Read the model definition and answer for the solid it produces. Units are mm, in the model's axes. A direction names the side the tool comes from. Round coordinates to 2 decimals unless told otherwise and drop trailing zeros. Use one line per item in the form item = value. Start each with the question number.
from build123d import *

# Parameters (mm, degrees)
F0_R          = 2.125
F0_R_2        = 5.25
F1_DEPTH      = 5
F3_DEPTH      = 15
F4_R          = 2.125
F5_DEPTH      = 25
F6_W          = 50
F6_H          = 15
F6_R          = 2.125
F7_DEPTH      = 5
F8_R          = 7.5
F9_SIZE       = 7.5
F10_R         = 2.125
F10_R_2       = 11.5
F11_DEPTH     = 3.75
F12_T1_DEPTH  = 10
F12_T6_DEPTH  = 4
F12_S7_R      = 25
F12_T8_DEPTH  = 4
F12_T12_DEPTH = 4
F12_S13_R     = 25
F12_T14_DEPTH = 4
F13_R         = 4.99999
F14_R         = 1.99999
F15_R         = 5.5
F16_DEPTH     = 25


# Not quite as in the source:
# - a fillet or chamfer that OpenCascade refuses, or shapes differently, is made with other operations: its cross-section is extruded or revolved along the edge and cut away or added
# - a fillet or chamfer is up to 0.001 mm smaller than in the source, because OpenCascade refuses the exact size


with BuildPart() as f1:
    # F0 (on Top) → F1 (new body)
    with BuildSketch(Plane.XY):
        with BuildLine():
            Line((25, -27.1), (25, -22.1))
            Line((25, -22.1), (25, 0))
            ThreePointArc((25, 0), (0, 25), (-25, 0))
            Line((-25, 0), (-25, -22.1))
            Line((-25, -22.1), (-25, -27.1))
            Line((-25, -27.1), (25, -27.1))
        make_face()
        with Locations((-13.8564064606, -8)):
            Circle(F0_R, mode=Mode.SUBTRACT)
        with Locations((13.8564064606, -8)):
            Circle(F0_R, mode=Mode.SUBTRACT)
        Circle(F0_R_2, mode=Mode.SUBTRACT)
        with Locations((0, 16)):
            Circle(F0_R, mode=Mode.SUBTRACT)
    extrude(amount=F1_DEPTH)

    # F2 (on face) → F3 (join)
    with BuildSketch(Plane.XY.offset(5)):
        Polygon((-25, -27.1), (25, -27.1), (25, -22.1), (25, 0), (21, 0), (21, -22.1), (5, -22.1), (5, -14.1), (0, -14.1), (-5, -14.1), (-5, -22.1), (-21, -22.1), (-21, 0), (-25, 0), (-25, -22.1), align=None)
    extrude(amount=F3_DEPTH)

    # F4 (on face) → F5 (cut)
    with BuildSketch(Plane.XZ.offset(27.1)):
        with Locations((-11.725, 12.5)):
            Circle(F4_R)
        with Locations((11.725, 12.5)):
            Circle(F4_R)
    extrude(amount=-F5_DEPTH, mode=Mode.SUBTRACT)

    # F6 (on Top) → F7 (join)
    with BuildSketch(Plane.XY):
        with Locations((0, -34.6)):
            Rectangle(F6_W, F6_H)
        with Locations((-17.5, -34.6)):
            Circle(F6_R, mode=Mode.SUBTRACT)
        with Locations((17.5, -34.6)):
            Circle(F6_R, mode=Mode.SUBTRACT)
    extrude(amount=F7_DEPTH)

    # F8
    f8_edges = [f1.edges().sort_by_distance(p)[0] for p in [
        (-25, -42.1, 2.5),
        (25, -42.1, 2.5),
    ]]
    fillet(f8_edges, radius=F8_R)

    # F9
    f9_edges = [f1.edges().sort_by_distance(p)[0] for p in [
        (0, -14.1, 20),
        (-23, 0, 20),
        (23, 0, 20),
    ]]
    chamfer(f9_edges, length=F9_SIZE)

    # F10 (on face) → F11 (join)
    with BuildSketch(Plane.XY.offset(5)):
        with BuildLine():
            Line((25, -22.1), (25, 0))
            ThreePointArc((25, 0), (0, 25), (-25, 0))
            Line((-25, 0), (-25, -22.1))
            Line((-25, -22.1), (25, -22.1))
        make_face()
        with Locations((-13.8564064606, -8)):
            Circle(F10_R, mode=Mode.SUBTRACT)
        Circle(F10_R_2, mode=Mode.SUBTRACT)
        with Locations((13.8564064606, -8)):
            Circle(F10_R, mode=Mode.SUBTRACT)
        with Locations((0, 16)):
            Circle(F10_R, mode=Mode.SUBTRACT)
    extrude(amount=F11_DEPTH)

    # F12: chamfer of 2.5 on 3 edges, made by hand

    # F12_s2 → F12_t1 (join)
    with BuildSketch(Plane.YZ.offset(-5)):
        with BuildLine():
            Line((-14.1707106781, 11.3207106781), (-11.5292893219, 8.6792893219))
            Line((-11.5292893219, 8.6792893219), (-11.5292893219, 8.6292893219))
            ThreePointArc((-11.5292893219, 8.6292893219), (-12.8146446609, 8.7), (-14.1, 8.7))
            Line((-14.1, 8.7), (-14.15, 8.75))
            ThreePointArc((-14.15, 8.75), (-14.15, 10.0353553391), (-14.2207106781, 11.3207106781))
            Line((-14.2207106781, 11.3207106781), (-14.1707106781, 11.3207106781))
        make_face()
    extrude(amount=F12_T1_DEPTH)


with BuildPart() as f12_tool4:
    # F12_s5 → F12_t6 (new body)
    with BuildSketch(Plane.YZ.offset(-21)):
        with BuildLine():
            Line((-0.0707106781, 11.3207106781), (2.5707106781, 8.6792893219))
            Line((2.5707106781, 8.6792893219), (2.5707106781, 8.6292893219))
            ThreePointArc((2.5707106781, 8.6292893219), (1.2853553391, 8.7), (0, 8.7))
            Line((0, 8.7), (-0.05, 8.75))
            ThreePointArc((-0.05, 8.75), (-0.05, 10.0353553391), (-0.1207106781, 11.3207106781))
            Line((-0.1207106781, 11.3207106781), (-0.0707106781, 11.3207106781))
        make_face()
    extrude(amount=-F12_T6_DEPTH)

    # F12_s7 → F12_t8 (intersect, symmetric)
    with BuildSketch(Plane.XY.offset(10)):
        Circle(F12_S7_R)
    extrude(amount=F12_T8_DEPTH, both=True, mode=Mode.INTERSECT)


with BuildPart() as f1_1:
    add(f1.part)

    # F12_t3: union F12_tool4
    add(f12_tool4.part)


with BuildPart() as f12_tool10:
    # F12_s11 → F12_t12 (new body)
    with BuildSketch(Plane.YZ.offset(25)):
        with BuildLine():
            Line((2.5707106781, 8.6792893219), (-0.0707106781, 11.3207106781))
            Line((-0.0707106781, 11.3207106781), (-0.1207106781, 11.3207106781))
            ThreePointArc((-0.1207106781, 11.3207106781), (-0.05, 10.0353553391), (-0.05, 8.75))
            Line((-0.05, 8.75), (0, 8.7))
            ThreePointArc((0, 8.7), (1.2853553391, 8.7), (2.5707106781, 8.6292893219))
            Line((2.5707106781, 8.6292893219), (2.5707106781, 8.6792893219))
        make_face()
    extrude(amount=-F12_T12_DEPTH)

    # F12_s13 → F12_t14 (intersect, symmetric)
    with BuildSketch(Plane.XY.offset(10)):
        Circle(F12_S13_R)
    extrude(amount=F12_T14_DEPTH, both=True, mode=Mode.INTERSECT)


with BuildPart() as f1_2:
    add(f1_1.part)

    # F12_t9: union F12_tool10
    add(f12_tool10.part)

    # F13 (radius 5 in the source; OpenCascade refuses exactly that, so slightly less here)
    f13_edges = [f1_2.edges().sort_by_distance(p)[0] for p in [
        (5, -17.85, 16.25),
        (-5, -17.85, 16.25),
    ]]
    fillet(f13_edges, radius=F13_R)

    # F14 (radius 2 in the source; OpenCascade refuses exactly that, so slightly less here)
    f14_edges = [f1_2.edges().sort_by_distance(p)[0] for p in [
        (21, -14.8, 20),
        (25, -17.3, 20),
        (-21, -14.8, 20),
        (-25, -17.3, 20),
        (0, 25, 8.75),
    ]]
    fillet(f14_edges, radius=F14_R)

    # F15 (on face) → F16 (cut)
    with BuildSketch(Plane.XY.offset(5)):
        Circle(F15_R)
    extrude(amount=-F16_DEPTH, mode=Mode.SUBTRACT)


solid = f1_2.part
Item 1: Find the intervals of material crossed by L1, parallel to Y at x = 0, z = 2.75 (3 decimals); L2, parallel to X at y = -9, z = 16.5; L3, parallel to Y at x = 0, z = 6 (3 decimals), in increasing order. Write a range as [from, to].
Item 2: For a pull along X with two mould halves and no side action, classify faces 1 (the cylindrical face through (22.861, -39.845, 2.535)), 2 (the flat face through (-3, -5, 5)), 3 (the flat face through (0, -42.1, 2)) as pulls with the +X half, pulls with the -X half, needs draft (parallel to the pull), parting line crosses it, or undercut.
Item 3: Given P1, Ø10, axis at x = -14, z = 8, coming from the +Y side; P2, Ø5, axis at x = -11.725, z = 12.5, coming from the -Y side; P3, Ø3.5, axis at x = -11, z = 16, coming from the +Y side, each flat-ended and moving along its own axis, determine where each tip first touches the part or whether it passes through.
Item 4: A tool of negligible diameter and unlimited length cuts with its end or side. For faces 4 (the cylindrical face through (24.4, -16.15, 19.43)), 5 (the flat face through (0, -34, 5)), 6 (the flat face through (13, -22.1, 16)), from which of +Z, -Z, +X, -X, +Y, -Y can it reach the whole face along a straight path? Write none if from no direction.
The answers:
q1.L1 = [-42.1, -5.5], [5.5, 13.875], [18.125, 25]
q1.L2 = [-25, -21], [21, 25]
q1.L3 = [-27.1, -11.5], [11.5, 13.875], [18.125, 25]
q2.face_1 = pulls with the +X half
q2.face_2 = undercut
q2.face_3 = needs draft
q3.P1 = 23.27
q3.P2 = -27.1
q3.P3 = -22.1
q4.face_4 = +Z, +X, +Y, -Y
q4.face_5 = +Z, +X, -X, -Y
q4.face_6 = +Z, +Y
